For this review, take the finished solid that the model builds, in its own axes (mm). A direction names the side the tool comes from. Coordinates: 2 decimals unless noted, no trailing zeros. Order: outer loops, then holes, each group sorted by start corner. A loop starts at its lowest first (then second) coordinate and runs counter-clockwise, first axis right, second up. Notation, with made-up numbers: (46.25, 59) -> (91.25, 59) arc R20 ccw to (91.25, 65) -> close; hole circle Ø11 at (-34, 25). An arc over 180 degrees is marked (long way). Return JSON: item names as keys, results as strings. Group by question number.
Item 1: Draft analysis for pull direction X (two halves, no side actions). For faces 4 (the conical face through (-7.26, 15.62, -23.04)), 5 (the conical face through (-16.178, 5.523, 16.22)), 6 (the cylindrical face through (16.4, 10.61, 16.45)), 7 (the conical face through (-0.694, 13.823, 1.673)), state which applies: +X half, -X half, draft (parallel to the pull), parting line (faces both ways), or undercut.
Item 2: Take a section at C-C (y = 18.5). Write out the cut boundary in (x, z).
Item 3: For line 1 along X through (y, z) = (6.75, -23); line 2 along X through (y, z) = (8.75, 4); line 3 along X through (y, z) = (16, 0), list the stretches that pass through material, from the lowest coordinate up.
Item 4: Machinability: for faces 1 (the cylindrical face through (-23.23, 10.61, -0.03)), 2 (the cylindrical face through (-16.45, 10.61, 16.4)), 3 (the cylindrical face through (-0.03, 10.61, 23.23)), which of the approach directions +Z, -Z, +X, -X, +Y, -Y give a long, thin tool a straight path to every point of the face, cutting with its end or side? Answer none if there is none.
Item 5: Insertion check: pin 1 (8 mm diameter, centred on y = 2, z = 0.5, fed in from -X); pin 2 (2 mm diameter, centred on y = 18.5, z = -2.5, fed in from -X); pin 3 (4 mm diameter, centred on x = 10, z = -27, fed in from -Y). Each pin has a flat end and moves straight along its axis. Give the tip position at first contact, or say it passes through.
```python
from build123d import *

# Parameters (mm, degrees)
SKETCH1_W          = 23.2283
SKETCH1_H          = 15.24
CUT_EXTRUDE1_START = -15.24
CUT_EXTRUDE1_DEPTH = 15.24
SKETCH3_R          = 1.6764
CUT_EXTRUDE2_DEPTH = 15.24
CUT_EXTRUDE3_START = -5.08
SKETCH4_R          = 23.2283
SKETCH4_R_2        = 22.5806
CUT_EXTRUDE3_DEPTH = 5.08
CHAMFER1_SIZE      = 0.762
DRAFT1_ANGLE       = 1


with BuildPart() as part:
    # Sketch1 → Revolve1 (revolve)
    with BuildSketch(Plane.XY, mode=Mode.PRIVATE) as revolve1_sk:
        with Locations((11.61415, 7.62)):
            Rectangle(SKETCH1_W, SKETCH1_H)
        Polygon((0, 21.336), (0, 15.24), (23.2283, 15.24), (38.1, 21.336), align=None)
    revolve(revolve1_sk.sketch.rotate(Axis((0, 0, 0), (0, 1, 0)), 90), axis=Axis((0, 0, 0), (0, 1, 0)))

    # Sketch2 → Cut-Extrude1 (cut)
    with BuildSketch(Plane.XZ.offset(CUT_EXTRUDE1_START)):
        with BuildLine():
            Line((2.159, 23.127746105), (2.09879825, 22.482849959))
            ThreePointArc((2.09879825, 22.482849959), (8.641221513, 20.861754172), (14.413701191, 17.381850141))
            Line((14.413701191, 17.381850141), (14.827142564, 17.880429645))
            ThreePointArc((14.827142564, 17.880429645), (8.889085572, 21.460150945), (2.159, 23.127746105))
        make_face()
        with BuildLine():
            ThreePointArc((-14.413701191, 17.381850141), (-8.641221513, 20.861754172), (-2.09879825, 22.482849959))
            Line((-2.09879825, 22.482849959), (-2.159, 23.127746105))
            ThreePointArc((-2.159, 23.127746105), (-8.889085572, 21.460150945), (-14.827142564, 17.880429645))
            Line((-14.827142564, 17.880429645), (-14.413701191, 17.381850141))
        make_face()
        with BuildLine():
            Line((-23.127746105, 2.159), (-22.482849959, 2.09879825))
            ThreePointArc((-22.482849959, 2.09879825), (-20.861754172, 8.641221513), (-17.381850141, 14.413701191))
            Line((-17.381850141, 14.413701191), (-17.880429645, 14.827142564))
            ThreePointArc((-17.880429645, 14.827142564), (-21.460150945, 8.889085572), (-23.127746105, 2.159))
        make_face()
        with BuildLine():
            Line((-17.880429645, -14.827142564), (-17.381850141, -14.413701191))
            ThreePointArc((-17.381850141, -14.413701191), (-20.861754172, -8.641221513), (-22.482849959, -2.09879825))
            Line((-22.482849959, -2.09879825), (-23.127746105, -2.159))
            ThreePointArc((-23.127746105, -2.159), (-21.460150945, -8.889085572), (-17.880429645, -14.827142564))
        make_face()
        with BuildLine():
            Line((-2.159, -23.127746105), (-2.09879825, -22.482849959))
            ThreePointArc((-2.09879825, -22.482849959), (-8.641221513, -20.861754172), (-14.413701191, -17.381850141))
            Line((-14.413701191, -17.381850141), (-14.827142564, -17.880429645))
            ThreePointArc((-14.827142564, -17.880429645), (-8.889085572, -21.460150945), (-2.159, -23.127746105))
        make_face()
        with BuildLine():
            Line((14.827142564, -17.880429645), (14.413701191, -17.381850141))
            ThreePointArc((14.413701191, -17.381850141), (8.641221513, -20.861754172), (2.09879825, -22.482849959))
            Line((2.09879825, -22.482849959), (2.159, -23.127746105))
            ThreePointArc((2.159, -23.127746105), (8.889085572, -21.460150945), (14.827142564, -17.880429645))
        make_face()
        with BuildLine():
            Line((23.127746105, -2.159), (22.482849959, -2.09879825))
            ThreePointArc((22.482849959, -2.09879825), (20.861754172, -8.641221513), (17.381850141, -14.413701191))
            Line((17.381850141, -14.413701191), (17.880429645, -14.827142564))
            ThreePointArc((17.880429645, -14.827142564), (21.460150945, -8.889085572), (23.127746105, -2.159))
        make_face()
        with BuildLine():
            Line((17.880429645, 14.827142564), (17.381850141, 14.413701191))
            ThreePointArc((17.381850141, 14.413701191), (20.861754172, 8.641221513), (22.482849959, 2.09879825))
            Line((22.482849959, 2.09879825), (23.127746105, 2.159))
            ThreePointArc((23.127746105, 2.159), (21.460150945, 8.889085572), (17.880429645, 14.827142564))
        make_face()
    extrude(amount=CUT_EXTRUDE1_DEPTH, mode=Mode.SUBTRACT)

    # Sketch3 → Cut-Extrude2 (cut)
    with BuildSketch(Plane(origin=(0, 21.336, 0), x_dir=(1, 0, 0), z_dir=(0, 1, 0))):
        with Locations(Location((0, 0, 0), (0, 0, 270))):
            Circle(SKETCH3_R)
    extrude(amount=-CUT_EXTRUDE2_DEPTH, mode=Mode.SUBTRACT)

    # Sketch4 → Cut-Extrude3 (cut)
    with BuildSketch(Plane.XZ.offset(CUT_EXTRUDE3_START)):
        Circle(SKETCH4_R)
        with Locations(Location((0, 0, 0), (0, 0, 270))):
            Circle(SKETCH4_R_2, mode=Mode.SUBTRACT)
    extrude(amount=CUT_EXTRUDE3_DEPTH, mode=Mode.SUBTRACT)

    # Chamfer1
    # the kernel refuses this chamfer: 0.762 mm, written as the material it takes off along each edge
    with BuildSketch(Plane(origin=(0, 5.08, 0), x_dir=(-0.17651563537313197, 0, -0.9842978362613723), z_dir=(-0.9842978362613723, 0, 0.17651563537313197))) as chamfer1_piece_1_section:
        Polygon((23.2283 - CHAMFER1_SIZE, 0), (23.2283, -CHAMFER1_SIZE), (23.2283, 0), align=None)
    chamfer1_piece_1 = revolve(axis=Axis((0, 5.08, 0), (0, -1, 0)), revolution_arc=20.333741592, mode=Mode.PRIVATE)
    chamfer1_piece_1 = chamfer1_piece_1 - Plane(origin=(0, 5.340057495, 0), x_dir=(0, 0, -1), z_dir=(0, 1, 0)) * Cylinder(22.5806, 93, mode=Mode.PRIVATE)
    add(chamfer1_piece_1, mode=Mode.SUBTRACT)
    with BuildSketch(Plane(origin=(0, 5.08, 0), x_dir=(0.5711882719698622, 0, -0.8208190774854607), z_dir=(-0.8208190774854607, 0, -0.5711882719698622))) as chamfer1_piece_2_section:
        Polygon((23.2283, -CHAMFER1_SIZE), (23.2283 - CHAMFER1_SIZE, 0), (23.2283, 0), align=None)
    chamfer1_piece_2 = revolve(axis=Axis((0, 5.08, 0), (0, -1, 0)), revolution_arc=20.333741592, mode=Mode.PRIVATE)
    chamfer1_piece_2 = chamfer1_piece_2 - Plane(origin=(0, 5.340057495, 0), x_dir=(0, 0, -1), z_dir=(0, 1, 0)) * Cylinder(22.5806, 93, mode=Mode.PRIVATE)
    add(chamfer1_piece_2, mode=Mode.SUBTRACT)
    with BuildSketch(Plane(origin=(0, 5.08, 0), x_dir=(0.9842978362613659, 0, -0.17651563537316883), z_dir=(-0.17651563537316883, 0, -0.9842978362613659))) as chamfer1_piece_3_section:
        Polygon((23.2283 - CHAMFER1_SIZE, 0), (23.2283, -CHAMFER1_SIZE), (23.2283, 0), align=None)
    chamfer1_piece_3 = revolve(axis=Axis((0, 5.08, 0), (0, -1, 0)), revolution_arc=20.333741592, mode=Mode.PRIVATE)
    chamfer1_piece_3 = chamfer1_piece_3 - Plane(origin=(0, 5.340057495, 0), x_dir=(0, 0, -1), z_dir=(0, 1, 0)) * Cylinder(22.5806, 93, mode=Mode.PRIVATE)
    add(chamfer1_piece_3, mode=Mode.SUBTRACT)
    with BuildSketch(Plane(origin=(0, 5.08, 0), x_dir=(0.8208190774854608, 0, 0.5711882719698618), z_dir=(0.5711882719698618, 0, -0.8208190774854608))) as chamfer1_piece_4_section:
        Polygon((23.2283 - CHAMFER1_SIZE, 0), (23.2283, -CHAMFER1_SIZE), (23.2283, 0), align=None)
    chamfer1_piece_4 = revolve(axis=Axis((0, 5.08, 0), (0, -1, 0)), revolution_arc=20.333741592, mode=Mode.PRIVATE)
    chamfer1_piece_4 = chamfer1_piece_4 - Plane(origin=(0, 5.340057495, 0), x_dir=(0, 0, -1), z_dir=(0, 1, 0)) * Cylinder(22.5806, 93, mode=Mode.PRIVATE)
    add(chamfer1_piece_4, mode=Mode.SUBTRACT)
    with BuildSketch(Plane(origin=(0, 5.08, 0), x_dir=(0.1765156353731264, 0, 0.9842978362613735), z_dir=(0.9842978362613735, 0, -0.1765156353731264))) as chamfer1_piece_5_section:
        Polygon((23.2283 - CHAMFER1_SIZE, 0), (23.2283, -CHAMFER1_SIZE), (23.2283, 0), align=None)
    chamfer1_piece_5 = revolve(axis=Axis((0, 5.08, 0), (0, -1, 0)), revolution_arc=20.333741592, mode=Mode.PRIVATE)
    chamfer1_piece_5 = chamfer1_piece_5 - Plane(origin=(0, 5.340057495, 0), x_dir=(0, 0, -1), z_dir=(0, 1, 0)) * Cylinder(22.5806, 93, mode=Mode.PRIVATE)
    add(chamfer1_piece_5, mode=Mode.SUBTRACT)
    with BuildSketch(Plane(origin=(0, 5.08, 0), x_dir=(-0.5711882719698653, 0, 0.8208190774854587), z_dir=(0.8208190774854587, 0, 0.5711882719698653))) as chamfer1_piece_6_section:
        Polygon((23.2283 - CHAMFER1_SIZE, 0), (23.2283, -CHAMFER1_SIZE), (23.2283, 0), align=None)
    chamfer1_piece_6 = revolve(axis=Axis((0, 5.08, 0), (0, -1, 0)), revolution_arc=20.333741592, mode=Mode.PRIVATE)
    chamfer1_piece_6 = chamfer1_piece_6 - Plane(origin=(0, 5.340057495, 0), x_dir=(0, 0, -1), z_dir=(0, 1, 0)) * Cylinder(22.5806, 93, mode=Mode.PRIVATE)
    add(chamfer1_piece_6, mode=Mode.SUBTRACT)
    with BuildSketch(Plane(origin=(0, 5.08, 0), x_dir=(-0.9842978362613705, 0, 0.17651563537314238), z_dir=(0.17651563537314238, 0, 0.9842978362613705))) as chamfer1_piece_7_section:
        Polygon((23.2283 - CHAMFER1_SIZE, 0), (23.2283, -CHAMFER1_SIZE), (23.2283, 0), align=None)
    chamfer1_piece_7 = revolve(axis=Axis((0, 5.08, 0), (0, -1, 0)), revolution_arc=20.333741592, mode=Mode.PRIVATE)
    chamfer1_piece_7 = chamfer1_piece_7 - Plane(origin=(0, 5.340057495, 0), x_dir=(0, 0, -1), z_dir=(0, 1, 0)) * Cylinder(22.5806, 93, mode=Mode.PRIVATE)
    add(chamfer1_piece_7, mode=Mode.SUBTRACT)
    with BuildSketch(Plane(origin=(0, 5.08, 0), x_dir=(-0.8208190774854607, 0, -0.5711882719698622), z_dir=(-0.5711882719698622, 0, 0.8208190774854607))) as chamfer1_piece_8_section:
        Polygon((23.2283 - CHAMFER1_SIZE, 0), (23.2283, -CHAMFER1_SIZE), (23.2283, 0), align=None)
    chamfer1_piece_8 = revolve(axis=Axis((0, 5.08, 0), (0, -1, 0)), revolution_arc=20.333741592, mode=Mode.PRIVATE)
    chamfer1_piece_8 = chamfer1_piece_8 - Plane(origin=(0, 5.340057495, 0), x_dir=(0, 0, -1), z_dir=(0, 1, 0)) * Cylinder(22.5806, 93, mode=Mode.PRIVATE)
    add(chamfer1_piece_8, mode=Mode.SUBTRACT)

    # Draft1
    draft1_faces = [part.faces().sort_by_distance(p)[0] for p in [
        (0, 13.716, -1.6764),
    ]]
    draft(draft1_faces, Plane.ZX.offset(6.096), DRAFT1_ANGLE)


solid = part.part
```
Findings below:
{
 "1": {"face 4": "parting line", "face 5": "-X half", "face 6": "+X half", "face 7": "undercut"},
 "2": {"outline": "circle Ø62.36 at (0, 0); hole circle Ø3.79 at (0, 0)"},
 "3": {"line 1": "x = -2.15 to 2.15", "line 2": "x = -22.22 to 22.22", "line 3": "x = -25.08 to -1.85, 1.85 to 25.08"},
 "4": {"face 1": "-X, -Y", "face 2": "+Z, -X, -Y", "face 3": "+Z, -Y"},
 "5": {"pin 1": "stops at x = -23.23", "pin 2": "stops at x = -33.53", "pin 3": "stops at y = 16.7"}
}
